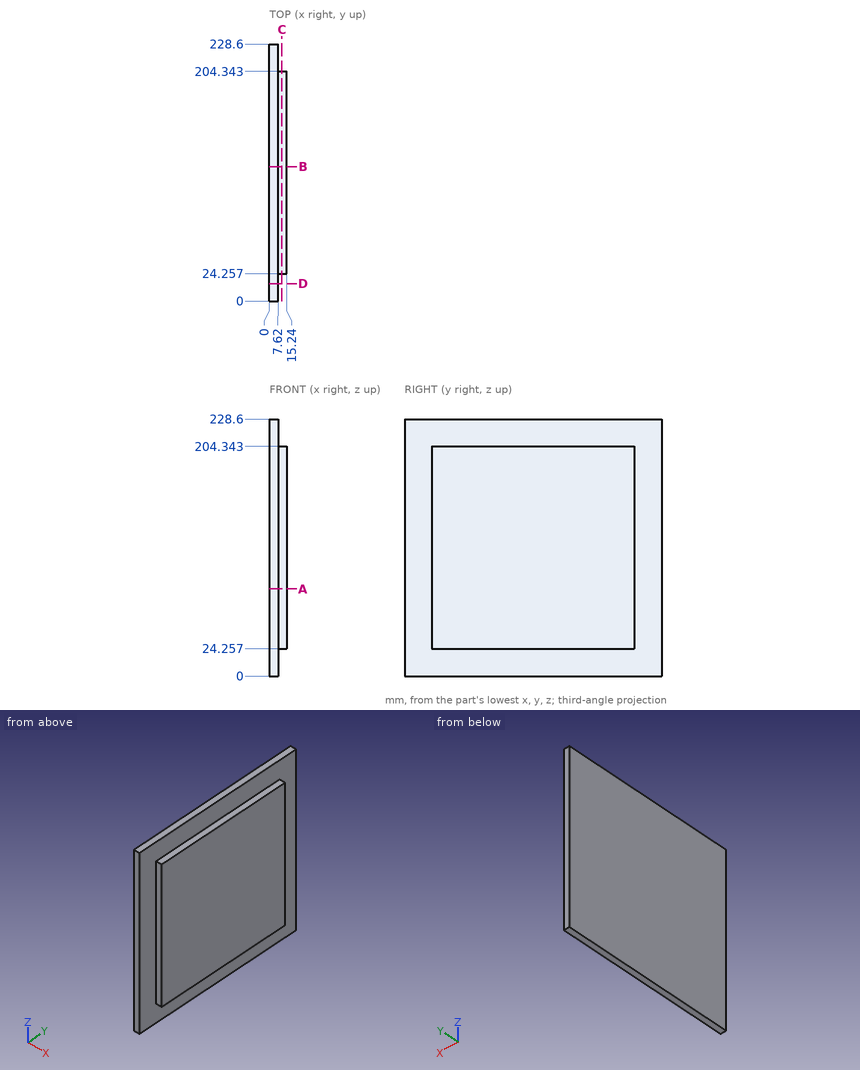
Source: three-view drawing plus pictorial views. Frame: mm from the lowest corner of the part. Give positions to 0.01 mm unless a question says otherwise; leave off trailing zeros. Order: outer loops, then holes, each group sorted by start corner. A loop starts at its lowest first (then second) coordinate and runs counter-clockwise, first axis right, second up. Notation, with made-up numbers: (64, 35.5) - (87, 35.5) arc R15 ccw to (87, 64.5) - close; hole circle Ø8 at (75, 61). An arc over 180 degrees is marked (long way). Answer as a JSON object with one key per item and string values. Group by question number.
Q1. Cut plane C-C, the plane x = 11. Output: boundary loops of the cut face in (y, z), then the cut area to 3 significant figures.
Q2. Line query: probe 1 along Y at (x, z) = (13.75, 45); probe 2 along X at (y, z) = (21.5, 31.5). Output: solid intervals per line, ascending.
Q3. First-contact query: pin 1 Ø5 at (x, z) = (9, 84) entering from +Y; pin 2 Ø4 at (x, z) = (11.5, 130.5) entering from +Y; pin 3 Ø2.5 at (x, y) = (12, 81.5) entering from +Z; pin 4 Ø6 at (x, z) = (12, 107.5) entering from -Y. Flat tips, straight axial feed; report the tip coordinate or a pass-through.
Q4. Cut plane A-A, the plane z = 77.5. Output: boundary loops of the cut face in (x, y).
Q5. Cut plane D-D, the plane y = 15.5. Output: boundary loops of the cut face in (x, z).
Results:
{
 "1": {"outline": "(24.26, 24.26) - (204.34, 24.26) - (204.34, 204.34) - (24.26, 204.34) - close", "area": "32,400 mm^2"},
 "2": {"probe 1": "24.26 to 204.34", "probe 2": "0 to 7.62"},
 "3": {"pin 1": "y = 228.6", "pin 2": "y = 204.34", "pin 3": "z = 204.34", "pin 4": "y = 24.26"},
 "4": {"outline": "(0, 0) - (7.62, 0) - (7.62, 24.26) - (15.24, 24.26) - (15.24, 204.34) - (7.62, 204.34) - (7.62, 228.6) - (0, 228.6) - close"},
 "5": {"outline": "(0, 0) - (7.62, 0) - (7.62, 228.6) - (0, 228.6) - close"}
}
